Geometry check sheet. Reference: drawing and pictorial views, mm from the part's lowest x, y, z. Coordinates: 2 decimals unless noted, no trailing zeros. Loops run counter-clockwise (first coordinate to the right, second up) from the corner with the lowest first, then second, coordinate; pieces in that order, holes last. Notation, with made-up numbers: (24.25, 10.25) -> (76.25, 10.25) arc R13 cw to (76.25, 29.25) -> close; hole circle Ø2 at (-18, -7). An arc over 180 degrees is marked (long way). Use one line per item in the form item = value.
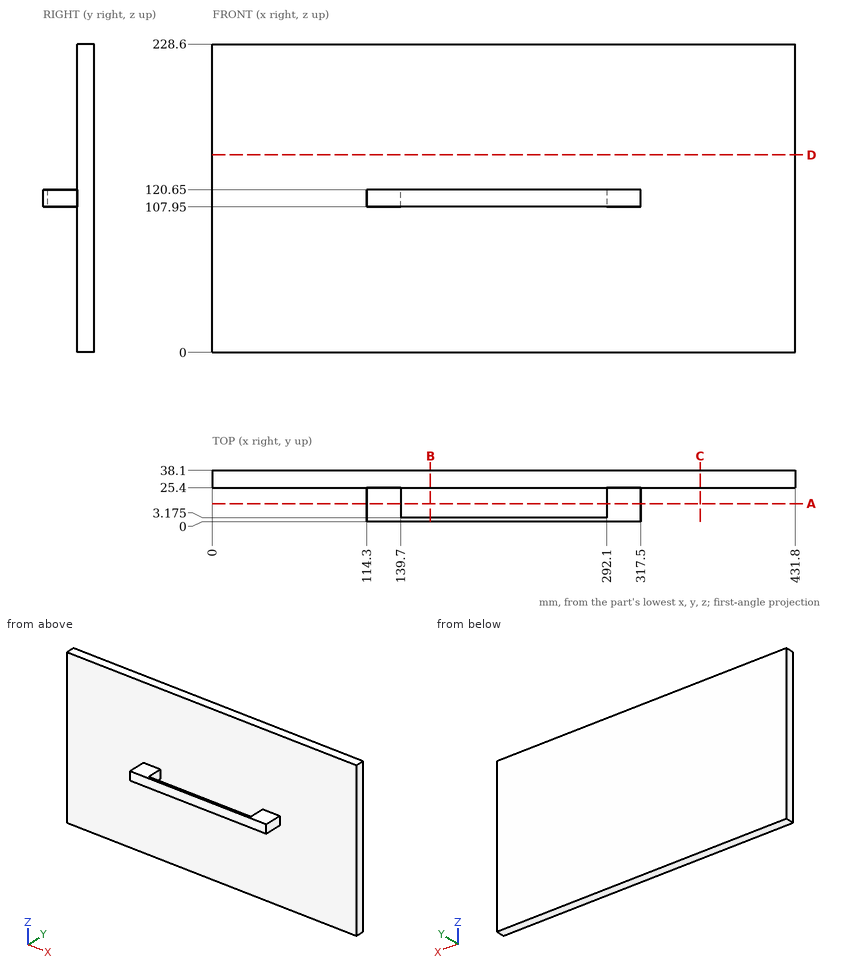
(1) Section check B-B, the plane x = 161.5. Record the boundary of the cut face in (y, z) (3 decimals).
Established:
outline = (0, 107.95) -> (3.175, 107.95) -> (3.175, 120.65) -> (0, 120.65) -> close; (25.4, 0) -> (38.1, 0) -> (38.1, 228.6) -> (25.4, 228.6) -> close
(2) Section check C-C, the plane x = 361.5. Record the boundary of the cut face in (y, z).
Established:
outline = (25.4, 0) -> (38.1, 0) -> (38.1, 228.6) -> (25.4, 228.6) -> close
(3) Section check D-D, the plane z = 146.5. Record the boundary of the cut face in (x, y), plus the area to 3 significant figures.
Established:
outline = (0, 25.4) -> (431.8, 25.4) -> (431.8, 38.1) -> (0, 38.1) -> close
area = 5,480 mm²
(4) Section check A-A, the plane y = 13.5. Record the boundary of the cut face in (x, z), plus the area to 3 significant figures.
Established:
outline = (114.3, 107.95) -> (139.7, 107.95) -> (139.7, 120.65) -> (114.3, 120.65) -> close; (292.1, 107.95) -> (317.5, 107.95) -> (317.5, 120.65) -> (292.1, 120.65) -> close
area = 645 mm²
(5) Scan lines: line 1 along X through (y, z) = (5, 116.5); line 2 along Y through (x, z) = (397, 11); line 3 along Z through (x, y) = (139, 15.5). Record each from-to range of solid material in increasing order.
Established:
line_1 = 114.3 to 139.7, 292.1 to 317.5
line_2 = 25.4 to 38.1
line_3 = 107.95 to 120.65
(6) Go/stop test with flat-tipped pins: P1, Ø4, axis at y = 18, z = 113, coming from the +X side; P2, Ø14, axis at y = 14, z = 116, coming from the -X side; P3, Ø1.5, axis at x = 252.5, z = 128.5, coming from the -Y side. Record where each tip stops, or that it passes through.
Established:
P1 = 317.5
P2 = 114.3
P3 = 25.4
